from build123d import *

# Parameters (mm, degrees)
EXTRUDE_1_DEPTH                = 5
SKETCH_2_R                     = 1.525
CUT_EXTRUDE_1_DEPTH            = 6
SKETCH_3_R                     = 48.25
EXTRUDE_2_DEPTH                = 5
SKETCH_4_R                     = 32
CUT_EXTRUDE_2_DEPTH            = 6
FILLET_1_R                     = 40
SKETCH_9_R                     = 7.5
CUT_EXTRUDE_7_DEPTH            = 6
SKETCH_10_R                    = 1.775
CUT_EXTRUDE_8_DEPTH            = 6
SKETCH_11_R                    = 1.525
CUT_EXTRUDE_9_DEPTH            = 6
SKETCH_15_R                    = 1.525
CUT_EXTRUDE_10_DEPTH           = 6
SKETCH_16_R                    = 1.525
SKETCH_16_R_2                  = 3.525
CUT_EXTRUDE_11_DEPTH           = 6
SKETCH_18_R                    = 1.525
CUT_EXTRUDE_13_DEPTH           = 6
CUT_EXTRUDE_14_DEPTH           = 6
FILLET_2_R                     = 2
PATTERN_LINEAR_1_COUNT         = 4
PATTERN_LINEAR_1_PITCH         = 35
FILLET_2_OF_PATTERN_LINEAR_1_R = 2


with BuildPart() as part:
    # 草图1 → 凸台-拉伸1 (new body)
    with BuildSketch(Plane(origin=(0, 0, 0), x_dir=(1, 0, 0), z_dir=(0, 1, 0))):
        with BuildLine():
            ThreePointArc((-78.875, 0), (-86.526835342, -18.473164658), (-105, -26.125))
            Line((-105, -26.125), (105, -26.125))
            Line((105, -26.125), (105, 26.125))
            Line((105, 26.125), (-105, 26.125))
            ThreePointArc((-105, 26.125), (-86.526835342, 18.473164658), (-78.875, 0))
        make_face()
        with BuildLine():
            ThreePointArc((-105, 26.125), (-131.125, 0), (-105, -26.125))
            Line((-105, -26.125), (-105, 26.125))
        make_face()
        with BuildLine():
            Line((-105, 26.125), (-105, -26.125))
            ThreePointArc((-105, -26.125), (-86.526835342, -18.473164658), (-78.875, 0))
            ThreePointArc((-78.875, 0), (-86.526835342, 18.473164658), (-105, 26.125))
        make_face()
    extrude(amount=EXTRUDE_1_DEPTH)

    # 草图2 → 切除-拉伸1 (cut, through all)
    with BuildSketch(Plane(origin=(0, 5, 0), x_dir=(1, 0, 0), z_dir=(0, 1, 0))):
        with Locations((-91.5, 0)):
            Circle(SKETCH_2_R)
        with Locations((-98.25, -11.691342951)):
            Circle(SKETCH_2_R)
        with Locations((-111.75, -11.691342951)):
            Circle(SKETCH_2_R)
        with Locations((-118.5, 0)):
            Circle(SKETCH_2_R)
        with Locations((-111.75, 11.691342951)):
            Circle(SKETCH_2_R)
        with Locations((-98.25, 11.691342951)):
            Circle(SKETCH_2_R)
    extrude(amount=-CUT_EXTRUDE_1_DEPTH, mode=Mode.SUBTRACT)

    # 草图3 → 凸台-拉伸2 (add)
    with BuildSketch(Plane(origin=(0, 5, 0), x_dir=(1, 0, 0), z_dir=(0, 1, 0))):
        with Locations((105, 0)):
            Circle(SKETCH_3_R)
    extrude(amount=-EXTRUDE_2_DEPTH)

    # 草图4 → 切除-拉伸2 (cut, through all)
    with BuildSketch(Plane(origin=(0, 5, 0), x_dir=(1, 0, 0), z_dir=(0, 1, 0))):
        with Locations((105, 0)):
            Circle(SKETCH_4_R)
    extrude(amount=-CUT_EXTRUDE_2_DEPTH, mode=Mode.SUBTRACT)

    # 圆角1
    fillet_1_edges = [part.edges().sort_by_distance(p)[0] for p in [
        (64.43465919, 2.5, 26.125),
        (64.43465919, 2.5, -26.125),
    ]]
    fillet(fillet_1_edges, radius=FILLET_1_R)

    # 草图9 → 切除-拉伸7 (cut, through all)
    with BuildSketch(Plane(origin=(0, 5, 0), x_dir=(1, 0, 0), z_dir=(0, 1, 0))):
        with Locations((-105, 0)):
            Circle(SKETCH_9_R)
    extrude(amount=-CUT_EXTRUDE_7_DEPTH, mode=Mode.SUBTRACT)

    # 草图10 → 切除-拉伸8 (cut, through all)
    with BuildSketch(Plane(origin=(0, 5, 0), x_dir=(1, 0, 0), z_dir=(0, 1, 0))):
        with Locations((73.533748237, 31.466251763)):
            Circle(SKETCH_10_R)
        with Locations((60.5, 0)):
            Circle(SKETCH_10_R)
        with Locations((73.533748237, -31.466251763)):
            Circle(SKETCH_10_R)
        with Locations((136.466251763, -31.466251763)):
            Circle(SKETCH_10_R)
        with Locations((136.466251763, 31.466251763)):
            Circle(SKETCH_10_R)
        with Locations((149.5, 0)):
            Circle(SKETCH_10_R)
        with Locations((105, -44.5)):
            Circle(SKETCH_10_R)
        with Locations((105, 44.5)):
            Circle(SKETCH_10_R)
    extrude(amount=-CUT_EXTRUDE_8_DEPTH, mode=Mode.SUBTRACT)

    # 草图11 → 切除-拉伸9 (cut, through all)
    with BuildSketch(Plane(origin=(0, 5, 0), x_dir=(1, 0, 0), z_dir=(0, 1, 0))):
        with Locations((122.02941274, 41.112639197)):
            Circle(SKETCH_11_R)
        with Locations((146.112639197, 17.02941274)):
            Circle(SKETCH_11_R)
        with Locations((146.112639197, -17.02941274)):
            Circle(SKETCH_11_R)
        with Locations((122.02941274, -41.112639197)):
            Circle(SKETCH_11_R)
        with Locations((87.97058726, -41.112639197)):
            Circle(SKETCH_11_R)
        with Locations((63.887360803, -17.02941274)):
            Circle(SKETCH_11_R)
        with Locations((63.887360803, 17.02941274)):
            Circle(SKETCH_11_R)
        with Locations((87.97058726, 41.112639197)):
            Circle(SKETCH_11_R)
    extrude(amount=-CUT_EXTRUDE_9_DEPTH, mode=Mode.SUBTRACT)

    # 草图15 → 切除-拉伸10 (cut, through all)
    with BuildSketch(Plane(origin=(0, 5, 0), x_dir=(1, 0, 0), z_dir=(0, 1, 0))):
        with Locations((-122.428761251, 10.0625)):
            Circle(SKETCH_15_R)
        with Locations((-105, 20.125)):
            Circle(SKETCH_15_R)
        with Locations((-87.571238749, 10.0625)):
            Circle(SKETCH_15_R)
        with Locations((-87.571238749, -10.0625)):
            Circle(SKETCH_15_R)
        with Locations((-105, -20.125)):
            Circle(SKETCH_15_R)
        with Locations((-122.428761251, -10.0625)):
            Circle(SKETCH_15_R)
    extrude(amount=-CUT_EXTRUDE_10_DEPTH, mode=Mode.SUBTRACT)

    # 草图16 → 切除-拉伸11 (cut, through all)
    with BuildSketch(Plane(origin=(0, 5, 0), x_dir=(1, 0, 0), z_dir=(0, 1, 0))):
        with Locations((-111.75, 11.691342951)):
            Circle(SKETCH_16_R)
        with Locations((-111.75, 11.691342951)):
            Circle(SKETCH_16_R_2)
        with Locations((-111.75, 11.691342951)):
            Circle(SKETCH_16_R, mode=Mode.SUBTRACT)
        with Locations((-98.25, 11.691342951)):
            Circle(SKETCH_16_R_2)
        with Locations((-98.25, 11.691342951)):
            Circle(SKETCH_16_R, mode=Mode.SUBTRACT)
        with Locations((-98.25, 11.691342951)):
            Circle(SKETCH_16_R)
        with Locations((-91.5, 0)):
            Circle(SKETCH_16_R)
        with Locations((-91.5, 0)):
            Circle(SKETCH_16_R_2)
        with Locations((-91.5, 0)):
            Circle(SKETCH_16_R, mode=Mode.SUBTRACT)
        with Locations((-98.25, -11.691342951)):
            Circle(SKETCH_16_R_2)
        with Locations((-98.25, -11.691342951)):
            Circle(SKETCH_16_R, mode=Mode.SUBTRACT)
        with Locations((-111.75, -11.691342951)):
            Circle(SKETCH_16_R_2)
        with Locations((-111.75, -11.691342951)):
            Circle(SKETCH_16_R, mode=Mode.SUBTRACT)
        with Locations((-111.75, -11.691342951)):
            Circle(SKETCH_16_R)
        with Locations((-118.5, 0)):
            Circle(SKETCH_16_R_2)
        with Locations((-118.5, 0)):
            Circle(SKETCH_16_R, mode=Mode.SUBTRACT)
        with Locations((-118.5, 0)):
            Circle(SKETCH_16_R)
    extrude(amount=-CUT_EXTRUDE_11_DEPTH, mode=Mode.SUBTRACT)

    # 草图18 → 切除-拉伸13 (cut, through all)
    with BuildSketch(Plane(origin=(0, 5, 0), x_dir=(1, 0, 0), z_dir=(0, 1, 0))):
        with Locations((45, 20.125)):
            Circle(SKETCH_18_R)
        with Locations((25, 20.125)):
            Circle(SKETCH_18_R)
        with Locations((5, 20.125)):
            Circle(SKETCH_18_R)
        with Locations((-15, 20.125)):
            Circle(SKETCH_18_R)
        with Locations((-35, 20.125)):
            Circle(SKETCH_18_R)
        with Locations((-55, 20.125)):
            Circle(SKETCH_18_R)
        with Locations((-75, 20.125)):
            Circle(SKETCH_18_R)
    cut_extrude_13 = extrude(amount=-CUT_EXTRUDE_13_DEPTH, mode=Mode.SUBTRACT)

    # 镜向1: 切除-拉伸13 across plane
    add(cut_extrude_13.mirror(Plane.XY), mode=Mode.SUBTRACT)

    # 草图19 → 切除-拉伸14 (cut, through all)
    with BuildSketch(Plane(origin=(0, 5, 0), x_dir=(1, 0, 0), z_dir=(0, 1, 0))):
        Polygon((-77, 14), (-77, -10.246335124), (-55.351486496, 14), align=None)
        Polygon((-52, 10.246335124), (-73.648513504, -14), (-52, -14), align=None)
    cut_extrude_14 = extrude(amount=-CUT_EXTRUDE_14_DEPTH, mode=Mode.SUBTRACT)

    # 圆角2
    fillet_2_edges = [part.edges().sort_by_distance(p)[0] for p in [
        (-52, 2.5, 14),
        (-73.648513504, 2.5, 14),
        (-52, 2.5, -10.246335124),
        (-77, 2.5, 10.246335124),
        (-77, 2.5, -14),
        (-55.351486496, 2.5, -14),
    ]]
    fillet(fillet_2_edges, radius=FILLET_2_R)

    # 阵列(线性)1: 切除-拉伸14 ×4
    with Locations(*[(i * PATTERN_LINEAR_1_PITCH, 0, 0) for i in range(1, PATTERN_LINEAR_1_COUNT)]):
        add(cut_extrude_14, mode=Mode.SUBTRACT)

    # 圆角2 of 阵列(线性)1
    fillet_2_of_pattern_linear_1_edges = [part.edges().sort_by_distance(p)[0] for p in [
        (-17, 2.5, 14),
        (-38.648513504, 2.5, 14),
        (-17, 2.5, -10.246335124),
        (-42, 2.5, 10.246335124),
        (-42, 2.5, -14),
        (-20.351486496, 2.5, -14),
        (18, 2.5, 14),
        (-3.648513504, 2.5, 14),
        (18, 2.5, -10.246335124),
        (-7, 2.5, 10.246335124),
        (-7, 2.5, -14),
        (14.648513504, 2.5, -14),
        (53, 2.5, 14),
        (31.351486496, 2.5, 14),
        (53, 2.5, -10.246335124),
        (28, 2.5, 10.246335124),
        (28, 2.5, -14),
        (49.648513504, 2.5, -14),
    ]]
    fillet(fillet_2_of_pattern_linear_1_edges, radius=FILLET_2_OF_PATTERN_LINEAR_1_R)


solid = part.part
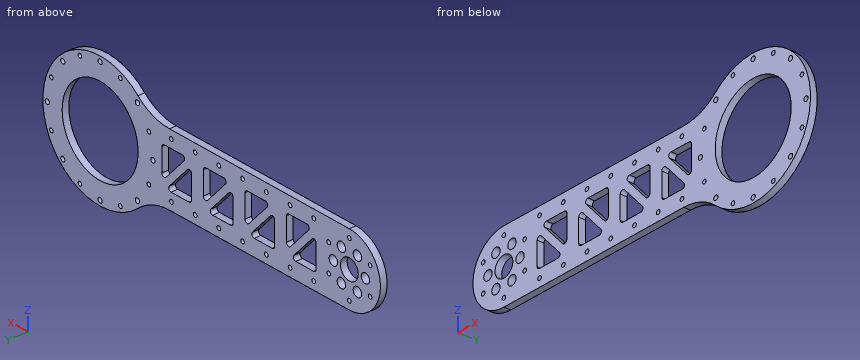
Input: part model. Units: mm. Frame: model coordinates. Give positions to 0.01 mm unless a question says otherwise; leave off trailing zeros. Loops run counter-clockwise (first coordinate to the right, second up) from the corner with the lowest first, then second, coordinate; pieces in that order, holes last. Notation, with made-up numbers: (28.25, 7) -> (55.25, 7) arc R22 ccw to (55.25, 20) -> close; hole circle Ø7 at (-40, 57.5). An arc over 180 degrees is marked (long way). Answer as a JSON object with one key per item and string values. Group by question number.
Item 1: Pin query (flat end, axial travel): P1, Ø1, axis at y = 1.5, z = -35.5, coming from the -X side; P2, Ø2.5, axis at x = -0.5, y = 3, coming from the +Z side (3 decimals); P3, Ø1.8, axis at x = 87.97, z = -41.11, coming from the -Y side. Return the tip coordinate at first contact, or that it passes through.
Item 2: Line query: probe 1 along Z at (x, y) = (-111.75, 3.1); probe 2 along Z at (x, y) = (-109.5, 2.25); probe 3 along Z at (x, y) = (9, 3) (3 decimals). Output: solid intervals per line, ascending.
Item 3: Cut plane C-C, the plane x = 56. Return the cut outline in (y, z).
Item 4: Cut plane B-B, the plane y = 2. State how many separate pieces and enclosed holes the cut face has, and give its area (3 significant figures).
Item 5: Cut plane A-A, the plane x = -29. Return the cut outline in (y, z) (3 decimals).
Checks:
{
 "1": {"P1": "stops at x = 71.68", "P2": "stops at z = 26.125", "P3": "passes through"},
 "2": {"probe 1": "z = -25.24 to -15.22, -8.17 to -3.27, 3.27 to 8.17, 15.22 to 25.24", "probe 2": "z = -25.73 to -14.4, -8.98 to -6, 6 to 8.98, 14.4 to 25.73", "probe 3": "z = -26.125 to -14, -7.674 to -0.166, 14 to 26.125"},
 "3": {"outline": "(0, -27.26) -> (5, -27.26) -> (5, 27.26) -> (0, 27.26) -> close"},
 "4": {"separate pieces": "1", "enclosed holes": "52", "area": "11,100 mm²"},
 "5": {"outline": "(0, -26.125) -> (5, -26.125) -> (5, -14) -> (0, -14) -> close; (0, -4.314) -> (5, -4.314) -> (5, 3.194) -> (0, 3.194) -> close; (0, 14) -> (5, 14) -> (5, 26.125) -> (0, 26.125) -> close"}
}
